Part model, mm, in its own coordinate system. A direction names the side the tool comes from. Round coordinates to 2 decimals unless told otherwise and drop trailing zeros. Write each loop counter-clockwise with the first axis right and the second up, starting at its lowest first coordinate (ties: lowest second). Pieces come first, ordered by that corner, then holes. Notation, with made-up numbers: M 36.25,83 L 57.25,83 A14 ccw 57.25,92 Z; hole C -40,16.5 d2. An arc over 180 degrees is marked long. Use a Markdown table: item, result. Add a question column.
1) Slice it at B-B on x = 30. Write the cut outline in (y, z).
2) Which spindle directions (+Z, -Z, +X, -X, +Y, -Y) get a long thin tool onto all of the face, cutting with end or side? Do faces 1 (the face through (85, 3, 1)), 2 (the face through (77, 10, 1)), 3 (the face through (12, -1, 1)). Say none if no direction does.
3) Slice it at A-A on y = 10.5. Write the cut outline in (x, z).
4) Wall check: probe 1 along X at (y, z) = (6.5, 2.9); probe 2 along X at (y, z) = (14.5, 0.35); probe 3 along Y at (x, z) = (79, 2.5). Give the ranges that are in metal, low to high.
5) Slice it at D-D on y = 4. Write the cut outline in (x, z), plus the area to 3 significant figures.
6) Slice it at C-C on z = 0.95. Give the number of separate pieces and of enclosed holes in the cut face, plus the area to 3 significant figures.
7) Drop flat-ended pins along their axis: P1, Ø0.9, axis at x = 9.5, z = 1, coming from the -Y side; P2, Ø0.9, axis at y = -2, z = 2, coming from the +X side. Give the stop position or say it passes through.
8) Two-plate mould, pull along X, no slides. Class faces 4 (the face through (76, -2, 1)), 5 (the face through (3, 4, 1)), 6 (the face through (9, 5, 1)): released by +X, released by -X, zero draft, split by the parting line, or undercut.
```python
from build123d import *

# Parameters (mm, degrees)
SKETCH_1_R      = 1.6
SKETCH_1_W      = 3
SKETCH_1_H      = 10
EXTRUDE_1_DEPTH = 3


with BuildPart() as part:
    # 草图1 → 凸台-拉伸1 (new body)
    with BuildSketch(Plane.XY):
        Polygon((3, 0), (12, 0), (12, -3), (32, -3), (32, 0), (56, 0), (56, -3), (76, -3), (76, 0), (85, 0), (85, 7), (88, 7), (88, 23), (85, 23), (85, 30), (3, 30), (3, 23), (0, 23), (0, 7), (3, 7), align=None)
        with Locations((30, 4)):
            Circle(SKETCH_1_R, mode=Mode.SUBTRACT)
        with Locations((58, 4)):
            Circle(SKETCH_1_R, mode=Mode.SUBTRACT)
        with Locations((9.5, 10)):
            Rectangle(SKETCH_1_W, SKETCH_1_H, mode=Mode.SUBTRACT)
        with Locations((78.5, 10)):
            Rectangle(SKETCH_1_W, SKETCH_1_H, mode=Mode.SUBTRACT)
    extrude(amount=EXTRUDE_1_DEPTH)


solid = part.part
```
Entries:
| question | item | result |
|---|---|---|
| 1 | outline | M -3,0 L 2.4,0 L 2.4,3 L -3,3 Z; M 5.6,0 L 30,0 L 30,3 L 5.6,3 Z |
| 2 | face 1 | +Z, -Z, +X, -Y |
| 2 | face 2 | +Z, -Z |
| 2 | face 3 | +Z, -Z, -X, -Y |
| 3 | outline | M 0,0 L 8,0 L 8,3 L 0,3 Z; M 11,0 L 77,0 L 77,3 L 11,3 Z; M 80,0 L 88,0 L 88,3 L 80,3 Z |
| 4 | probe 1 | x = 3 to 8, 11 to 77, 80 to 85 |
| 4 | probe 2 | x = 0 to 8, 11 to 77, 80 to 88 |
| 4 | probe 3 | y = 0 to 5, 15 to 30 |
| 5 | outline | M 3,0 L 28.4,0 L 28.4,3 L 3,3 Z; M 31.6,0 L 56.4,0 L 56.4,3 L 31.6,3 Z; M 59.6,0 L 85,0 L 85,3 L 59.6,3 Z |
| 5 | area | 227 mm^2 |
| 6 | separate pieces | 1 |
| 6 | enclosed holes | 4 |
| 6 | area | 2,600 mm^2 |
| 7 | P1 | stops at y = 0 |
| 7 | P2 | stops at x = 76 |
| 8 | face 4 | released by +X |
| 8 | face 5 | released by -X |
| 8 | face 6 | undercut |
